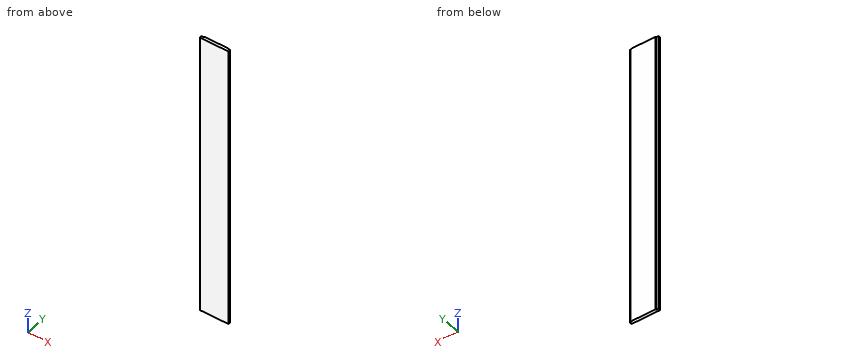
Autodesk Inventor part; units mm, degrees
ref_plane "YZ Plane" through (0, 0, 0) normal (1, 0, 0) x (0, 1, 0)
ref_plane "XZ Plane" through (0, 0, 0) normal (0, 1, 0) x (-1, 0, 0)
ref_plane "XY Plane" through (0, 0, 0) normal (0, 0, 1) x (1, 0, 0)
sketch "Sketch1" plane through (0, 0, 0) normal (0, 1, 0) x (-1, 0, 0)
  line L0 (135.7143, 497.619) -> (39.7143, 497.619)
  line L1 (39.7143, 497.619) -> (39.7143, -442.381)
  line L2 (39.7143, -442.381) -> (135.7143, -442.381)
  line L3 (135.7143, -442.381) -> (135.7143, 497.619)
  point P0 (0, 0)
  dimension "d0" = 940
  dimension "d1" = 96
extrude "Extrusion1" add sketch "Sketch1" along normal blind 14
sketch "Sketch2" plane through (-135.7143, 0, 497.619) normal (0, 0, 1) x (1, 0, 0)
  point P0 (135.7143, 0)
sketch "Sketch3" plane through (-135.7143, 0, 497.619) normal (0, 0, 1) x (1, 0, 0)
  line L0 (96, 14) -> (0, 14)
  line L1 (0, 14) -> (8, 14)
  line L2 (8, 14) -> (8, 8)
  line L3 (8, 8) -> (0, 8)
  line L4 (0, 8) -> (0, 14)
  line L5 (96, 14) -> (88, 14)
  line L6 (88, 14) -> (88, 8)
  line L7 (88, 8) -> (96, 8)
  line L8 (96, 8) -> (96, 14)
  line L9 (8, 14) -> (88, 14)
  line L10 (88, 14) -> (88, 10)
  line L11 (88, 10) -> (8, 10)
  line L12 (8, 10) -> (8, 14)
  point P0 (135.7143, 0)
  point P1 (8, 10)
  dimension "d4" = 8
  dimension "d5" = 6
  dimension "d6" = 6
extrude "Extrusion2" cut sketch "Sketch3" against normal through all
properties part number "TopZakrivka" material "Aluminum 6061"
Could you check a few things on this model? Use its own coordinates, in mm. Give positions to 0.01 mm unless a question says otherwise; leave off trailing zeros. Order: outer loops, then holes, each group sorted by start corner. A loop starts at its lowest first (then second) coordinate and runs counter-clockwise, first axis right, second up. Notation, with made-up numbers: (49.5, 85.25) -> (91.5, 85.25) arc R27 cw to (91.5, 102.25) -> close; hole circle Ø8 at (86.25, 16). An arc over 180 degrees is marked (long way). Answer in a Markdown table with one row per item. Add a question column.
Item 1: Please list where these lines run through material, in increasing order: probe 1 along Y at (x, z) = (-128, 166); probe 2 along X at (y, z) = (9, -141).
Item 2: I'm going to push flat-ended pins straight in: P1, Ø2.5, axis at x = -42, z = -175, coming from the +Y side; P2, Ø1.6, axis at y = 9, z = -110.5, coming from the -X side; P3, Ø0.6, axis at y = 9.5, z = 41.5, coming from the +X side. Where does each tip first touch, or does it pass through?
Item 3: Imagine slicing it at A-A (z = -292). List the corners of the cut face in (x, y) for me, and give its area (3 significant figures).
Result:
| question | item | result |
|---|---|---|
| 1 | probe 1 | 0 to 8 |
| 1 | probe 2 | -127.71 to -47.71 |
| 2 | P1 | y = 8 |
| 2 | P2 | x = -127.71 |
| 2 | P3 | x = -47.71 |
| 3 | outline | (-135.71, 0) -> (-39.71, 0) -> (-39.71, 8) -> (-47.71, 8) -> (-47.71, 10) -> (-127.71, 10) -> (-127.71, 8) -> (-135.71, 8) -> close |
| 3 | area | 928 mm2 |
